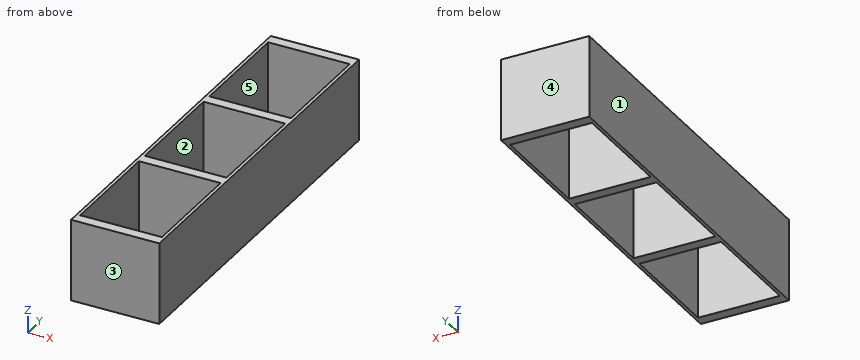
from build123d import *

# Parameters (mm, degrees)
SKETCH3_W           = 75
SKETCH3_H           = 75
BOSS_EXTRUDE2_DEPTH = 10
LPATTERN1_COUNT     = 4
LPATTERN1_PITCH     = 110
SKETCH3_5_W         = 3
SKETCH3_5_H         = 75
BOSS_EXTRUDE5_DEPTH = 340


with BuildPart() as part:
    # Sketch3 → Boss-Extrude2 (new body)
    with BuildSketch(Plane(origin=(0, 0, 0), x_dir=(1, 0, 0), z_dir=(0, 1, 0))):
        Rectangle(SKETCH3_W, SKETCH3_H)
    extrude(amount=BOSS_EXTRUDE2_DEPTH)


with BuildPart() as lpattern1_1:
    # LPattern1: pattern copy
    add(part.part.moved(Location(Vector(0, 1, 0) * (1 * LPATTERN1_PITCH))))


with BuildPart() as lpattern1_2:
    # LPattern1: pattern copy
    add(part.part.moved(Location(Vector(0, 1, 0) * (2 * LPATTERN1_PITCH))))


with BuildPart() as lpattern1_3:
    # LPattern1: pattern copy
    add(part.part.moved(Location(Vector(0, 1, 0) * (3 * LPATTERN1_PITCH))))


with BuildPart() as part_1:
    add(part.part)

    add(lpattern1_1.part)  # Boss-Extrude5 merges LPattern1_1

    add(lpattern1_2.part)  # Boss-Extrude5 merges LPattern1_2

    add(lpattern1_3.part)  # Boss-Extrude5 merges LPattern1_3
    # Sketch3<5> → Boss-Extrude5 (add)
    with BuildSketch(Plane(origin=(0, 0, 0), x_dir=(1, 0, 0), z_dir=(0, 1, 0))):
        with Locations((39, 0)):
            Rectangle(SKETCH3_5_W, SKETCH3_5_H)
        with Locations((-39, 0)):
            Rectangle(SKETCH3_5_W, SKETCH3_5_H)
    extrude(amount=BOSS_EXTRUDE5_DEPTH)


solid = part_1.part
CAD build for the part. Positions are in the model's coordinates, mm. Face numbers are marked on the shaded views. A direction names the side the tool comes from. Give positions to 0.01 mm unless a question says otherwise; leave off trailing zeros. Loops run counter-clockwise (first coordinate to the right, second up) from the corner with the lowest first, then second, coordinate; pieces in that order, holes last. Notation, with made-up numbers: M -40,44.25 L -30,44.25 A19 cw -30,56.25 Z; hole C -18.75,87 d4. An arc over 180 degrees is marked long. Answer in a Markdown table with one row per item. Add a question column.
Item 1: Tool access for the marked faces 4 and 5: list every direction of +Z, -Z, +X, -X, +Y, -Y with a clear straight run to the whole face (end or side of a thin tool).
Item 2: Band-saw the part on B-B on y = 283. Give the cut face in (x, z), then the cut area to 3 significant figures.
Item 3: Band-saw the part on A-A on x = -32. Give the cut face in (y, z), then the cut area to 3 significant figures.
Item 4: Probe probe 1 along Y at (x, z) = (12.5, 18.5); probe 2 along X at (y, z) = (156.5, 30). List the from-to ranges inside material, lowest first.
Item 5: Band-saw the part on C-C on z = -7.5. Give the cut face in (x, y).
Item 6: Drop a flat-ended pin along its axis: P1, Ø10, axis at x = -30, y = 74.5, coming from the +Z side. Give the stop position or say it passes through.
Item 7: Mould opens along X. For the marked faces 1, 2 and 3 say: +X half, -X half, draft (parallel to the pull), parting line (faces both ways), or undercut.
Reply:
| question | item | result |
|---|---|---|
| 1 | face 4 | +Z, -Z, +X, -X, +Y |
| 1 | face 5 | +Z, -Z |
| 2 | outline | M -40.5,-37.5 L -37.5,-37.5 L -37.5,37.5 L -40.5,37.5 Z; M 37.5,-37.5 L 40.5,-37.5 L 40.5,37.5 L 37.5,37.5 Z |
| 2 | area | 450 mm^2 |
| 3 | outline | M 0,-37.5 L 10,-37.5 L 10,37.5 L 0,37.5 Z; M 110,-37.5 L 120,-37.5 L 120,37.5 L 110,37.5 Z; M 220,-37.5 L 230,-37.5 L 230,37.5 L 220,37.5 Z; M 330,-37.5 L 340,-37.5 L 340,37.5 L 330,37.5 Z |
| 3 | area | 3,000 mm^2 |
| 4 | probe 1 | y = 0 to 10, 110 to 120, 220 to 230, 330 to 340 |
| 4 | probe 2 | x = -40.5 to -37.5, 37.5 to 40.5 |
| 5 | outline | M -40.5,0 L 40.5,0 L 40.5,340 L -40.5,340 Z; hole M -37.5,10 L 37.5,10 L 37.5,110 L -37.5,110 Z; hole M -37.5,120 L 37.5,120 L 37.5,220 L -37.5,220 Z; hole M -37.5,230 L 37.5,230 L 37.5,330 L -37.5,330 Z |
| 6 | P1 | passes through |
| 7 | face 1 | -X half |
| 7 | face 2 | undercut |
| 7 | face 3 | draft |
